CAD build for the part. Positions are in the model's coordinates, mm. Face numbers are marked on the shaded views. A direction names the side the tool comes from. Give positions to 0.01 mm unless a question says otherwise; leave off trailing zeros. Order: outer loops, then holes, each group sorted by start corner. A loop starts at its lowest first (then second) coordinate and runs counter-clockwise, first axis right, second up. Notation, with made-up numbers: (28.25, -31) -> (35.25, -31) arc R7 ccw to (35.25, -21) -> close; hole circle Ø1 at (-32.5, 59). An arc over 180 degrees is marked (long way). Use one line per item in the form item = value. Start each with the question number.
1) Probe line 1 (Z direction, x = 0, y = 3.25); line 2 (X direction, y = 6, z = 25); line 3 (Z direction, x = -3, y = 6.5). List the from-to ranges inside material, lowest first.
2) Cut at A-A, the plane x = 0. Give the cut face in (y, z) (3 decimals), and give its area (3 significant figures).
3) Tool access for the marked faces 5, 6 and 7: list every direction of +Z, -Z, +X, -X, +Y, -Y with a clear straight run to the whole face (end or side of a thin tool).
4) Cut at C-C, the plane y = 5. Give the cut face in (x, z), and give its area (3 significant figures).
5) Drop flat-ended pins along their axis: P1, Ø11.5, axis at x = 0, z = -25.4, coming from the +Y side (3 decimals); P2, Ø6.5, axis at x = 4, y = 20.5, coming from the -Z side; P3, Ø12, axis at y = 17.5, z = -16.5, coming from the -X side; P4, Ø12, axis at y = 24.5, z = -24, coming from the -X side. Give the stop position or say it passes through.
6) Cut at D-D, the plane z = 14. Give the cut face in (x, y) (3 decimals).
7) Cut at B-B, the plane z = 25.4. Give the cut face in (x, y) (3 decimals), and give its area (3 significant figures).
8) Mould opens along Z. For the marked faces 1, 2, 3 and 4 say: pulls with the +Z half, pulls with the -Z half, needs draft (parallel to the pull), parting line crosses it, or undercut.
from build123d import *

# Parameters (mm, degrees)
BOSS_EXTRUDE1_DEPTH     = 38.1
CUT_EXTRUDE2_DEPTH      = 25.4
F_3_8_CLEARANCE_HOLE2_D = 9.8044


with BuildPart() as part:
    # Sketch1 → Boss-Extrude1 (new, symmetric)
    with BuildSketch(Plane.XY):
        Polygon((0, 0), (25.4, 0), (25.4, 9.525), (3.175, 31.75), (-3.175, 31.75), (-25.4, 9.525), (-25.4, 0), align=None)
    extrude(amount=BOSS_EXTRUDE1_DEPTH, both=True)

    # Sketch6 → Cut-Extrude2 (cut)
    with BuildSketch(Plane.XY.offset(38.1)):
        Polygon((-25.4, 9.525), (25.4, 9.525), (3.175, 31.75), (-3.175, 31.75), align=None)
    cut_extrude2 = extrude(amount=-CUT_EXTRUDE2_DEPTH, mode=Mode.SUBTRACT)

    # 3/8 Clearance Hole2 (through all)
    with Locations(Plane(origin=(0, 9.525, 0), x_dir=(1, 0, 0), z_dir=(0, 1, 0))):
        with Locations((0, -25.4)):
            f_3_8_clearance_hole2 = Hole(F_3_8_CLEARANCE_HOLE2_D / 2)

    # Mirror2: Cut-Extrude2, 3/8 Clearance Hole2 across plane
    add(cut_extrude2.mirror(Plane.XY), mode=Mode.SUBTRACT)
    add(f_3_8_clearance_hole2.mirror(Plane.XY), mode=Mode.SUBTRACT)


solid = part.part
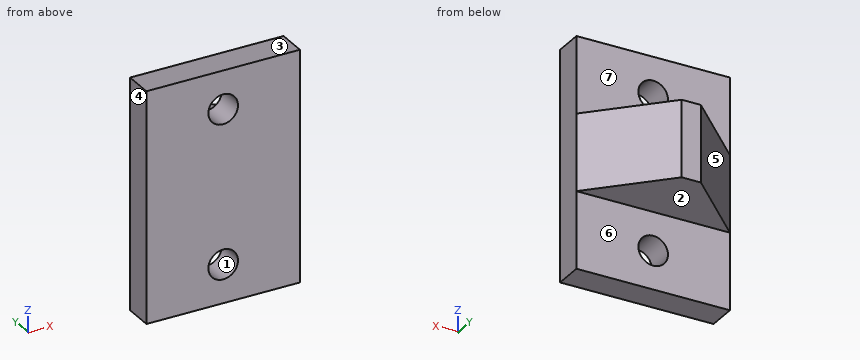
Result:
q1.line_1 = -38.1 to -30.3, -20.5 to 20.5, 30.3 to 38.1
q1.line_2 = -25.4 to -4.89, 4.89 to 25.4
q1.line_3 = -38.1 to -29.28, -21.52 to 21.52, 29.28 to 38.1
q2.outline = (0, -38.1) -> (9.525, -38.1) -> (9.525, -30.302) -> (0, -30.302) -> close; (0, -20.498) -> (9.525, -20.498) -> (9.525, -12.7) -> (31.75, -12.7) -> (31.75, 12.7) -> (9.525, 12.7) -> (9.525, 20.498) -> (0, 20.498) -> close; (0, 30.302) -> (9.525, 30.302) -> (9.525, 38.1) -> (0, 38.1) -> close
q2.area = 1,100 mm²
q3.face_5 = +Z, -Z, -X, +Y
q3.face_6 = -Z, +X, -X, +Y
q3.face_7 = +Z, +X, -X, +Y
q4.outline = (-25.4, -38.1) -> (25.4, -38.1) -> (25.4, 38.1) -> (-25.4, 38.1) -> close; hole circle Ø9.8 at (0, -25.4); hole circle Ø9.8 at (0, 25.4)
q4.area = 3,720 mm²
q5.P1 = 9.525
q5.P2 = -12.7
q5.P3 = -22.07
q5.P4 = through
q6.outline = (-25.4, 0) -> (25.4, 0) -> (25.4, 9.525) -> (-25.4, 9.525) -> close
q7.outline = (-25.4, 0) -> (-4.902, 0) -> (-4.902, 9.525) -> (-25.4, 9.525) -> close; (4.902, 0) -> (25.4, 0) -> (25.4, 9.525) -> (4.902, 9.525) -> close
q7.area = 390 mm²
q8.face_1 = undercut
q8.face_2 = pulls with the -Z half
q8.face_3 = pulls with the +Z half
q8.face_4 = needs draft
